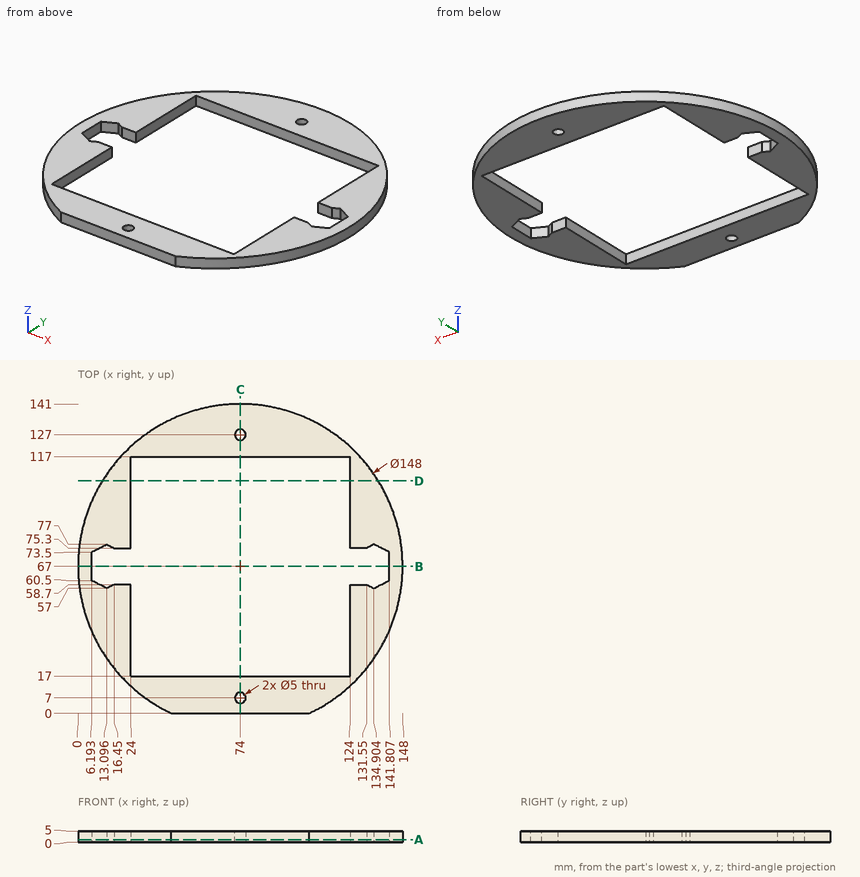
Could you check a few things on this drawing? It's one solid part, dimensions in mm from its lowest x, y, z. Round coordinates to 2 decimals unless told otherwise and drop trailing zeros. Order: outer loops, then holes, each group sorted by start corner. A loop starts at its lowest first (then second) coordinate and runs counter-clockwise, first axis right, second up. Notation, with made-up numbers: (89, 34) -> (122, 34) arc R17 cw to (122, 51) -> close; hole circle Ø8 at (-24.5, 3). An arc over 180 degrees is marked (long way). One line per question, with ' | ' between items.
Q1. If I drill on line 1 (Y direction, x = 74, z = 3.2); line 2 (X direction, y = 68, z = 3.1); line 3 (Y direction, x = 20.5, z = 1.55) (1 decimal), over which ranges is the centre line in solid material (lowest first)? Write a range as from..to.
Computed values:
line 1: 0..4.5, 9.5..17, 117..124.5, 129.5..141 | line 2: 0.01..6.19, 141.81..147.99 | line 3: 15.9..58.7, 75.3..118.1
Q2. If we section it at C-C on x = 74: Write out the boundary of the cut face in (y, z), plus the area to 3 significant figures.
Computed values:
outline: (0, 0) -> (4.5, 0) -> (4.5, 5) -> (0, 5) -> close; (9.5, 0) -> (17, 0) -> (17, 5) -> (9.5, 5) -> close; (117, 0) -> (124.5, 0) -> (124.5, 5) -> (117, 5) -> close; (129.5, 0) -> (141, 0) -> (141, 5) -> (129.5, 5) -> close | area: 155 mm²
Q3. If we section it at D-D on y = 106: Write out the boundary of the cut face in (x, z).
Computed values:
outline: (11.11, 0) -> (24, 0) -> (24, 5) -> (11.11, 5) -> close; (124, 0) -> (136.89, 0) -> (136.89, 5) -> (124, 5) -> close
Q4. If we section it at A-A on z = 1.2: Write out the boundary of the cut face in (x, y).
Computed values:
outline: (42.58, 0) -> (105.42, 0) arc R74 ccw (long way) to start; hole (6.19, 60.5) -> (13.1, 57) -> (16.45, 58.7) -> (24, 58.7) -> (24, 17) -> (124, 17) -> (124, 58.7) -> (131.55, 58.7) -> (134.9, 57) -> (141.81, 60.5) -> (141.81, 73.5) -> (134.9, 77) -> (131.55, 75.3) -> (124, 75.3) -> (124, 117) -> (24, 117) -> (24, 75.3) -> (16.45, 75.3) -> (13.1, 77) -> (6.19, 73.5) -> close; hole circle Ø5 at (74, 7); hole circle Ø5 at (74, 127)
Q5. I'm going to push flat-ended pins straight in: pin 1 (2.5 mm diameter, centred on x = 65, z = 3, fed in from +Y); pin 2 (2.5 mm diameter, centred on y = 96.5, z = 2.5, fed in from -X) (1 decimal); pin 3 (2 mm diameter, centred on y = 48, z = 3.5, fed in from -X); pin 4 (6.5 mm diameter, centred on x = 74, y = 7, fed in from +Z). Where does each tip first touch, or does it pass through?
Computed values:
pin 1: y = 140.59 | pin 2: x = 5.6 | pin 3: x = 2.22 | pin 4: z = 5
Q6. If we section it at B-B on y = 67: Write out the boundary of the cut face in (x, z).
Computed values:
outline: (0, 0) -> (6.19, 0) -> (6.19, 5) -> (0, 5) -> close; (141.81, 0) -> (148, 0) -> (148, 5) -> (141.81, 5) -> close
